Could you check a few things on this model? Use its own coordinates, in mm. Round coordinates to 2 decimals unless told otherwise and drop trailing zeros. Loops run counter-clockwise (first coordinate to the right, second up) from the corner with the lowest first, then second, coordinate; pieces in that order, holes last. Notation, with made-up numbers: (83, 4) -> (133, 4) arc R18 ccw to (133, 25) -> close; hole circle Ø6 at (-39, -39). An arc over 180 degrees is marked (long way). One line per item, written item: value.
```python
from build123d import *

# Parameters (mm, degrees)
BOSS_EXTRUDE1_DEPTH     = 1.5875
SKETCH2_R               = 0.635
CUT_EXTRUDE1_DEPTH      = 1
CUT_EXTRUDE1_DEPTH_BACK = 2.5875


with BuildPart() as part:
    # Sketch1 → Boss-Extrude1 (new body)
    with BuildSketch(Plane(origin=(0, 0, 0), x_dir=(1, 0, 0), z_dir=(0, 1, 0))):
        with BuildLine():
            Line((8.89, -66.675), (43.815, -66.675))
            Line((43.815, -66.675), (43.815, -1.27))
            ThreePointArc((43.815, -1.27), (43.453523156, -0.361476844), (42.545, 0))
            Line((42.545, 0), (-42.545, 0))
            Line((-42.545, 0), (-42.545, -57.785))
            Line((-42.545, -57.785), (-5.08, -57.785))
            ThreePointArc((-5.08, -57.785), (-4.181974388, -58.156974388), (-3.81, -59.055))
            ThreePointArc((-3.81, -59.055), (-3.438025612, -59.953025612), (-2.54, -60.325))
            Line((-2.54, -60.325), (2.54, -60.325))
            Line((2.54, -60.325), (2.54, -73.025))
            ThreePointArc((2.54, -73.025), (4.399871939, -68.534871939), (8.89, -66.675))
        make_face()
    extrude(amount=BOSS_EXTRUDE1_DEPTH)

    # Sketch2 → Cut-Extrude1 (cut, two sides)
    with BuildSketch(Plane(origin=(0, 1.5875, 0), x_dir=(-1, 0, 0), z_dir=(0, 1, 0))) as cut_extrude1_sk:
        with Locations((39.37, 3.175)):
            Circle(SKETCH2_R)
        with Locations((26.035, 3.175)):
            Circle(SKETCH2_R)
        with Locations((12.7, 3.175)):
            Circle(SKETCH2_R)
        with Locations((-0.635, 3.175)):
            Circle(SKETCH2_R)
        with Locations((-13.97, 3.175)):
            Circle(SKETCH2_R)
        with Locations((-27.305, 3.175)):
            Circle(SKETCH2_R)
        with Locations((-40.64, 3.175)):
            Circle(SKETCH2_R)
        with Locations((39.37, 16.03375)):
            Circle(SKETCH2_R)
        with Locations((39.37, 28.8925)):
            Circle(SKETCH2_R)
        with Locations((39.37, 41.75125)):
            Circle(SKETCH2_R)
        with Locations((-40.64, 15.24)):
            Circle(SKETCH2_R)
        with Locations((-40.64, 27.305)):
            Circle(SKETCH2_R)
        with Locations((-40.64, 39.37)):
            Circle(SKETCH2_R)
        with Locations((-40.64, 51.435)):
            Circle(SKETCH2_R)
        with Locations((-40.64, 63.5)):
            Circle(SKETCH2_R)
        with Locations((-24.994404736, 63.5)):
            Circle(SKETCH2_R)
        with Locations((-9.348809473, 63.5)):
            Circle(SKETCH2_R)
        with Locations((-1.889213751, 54.61)):
            Circle(SKETCH2_R)
        with Locations((11.863857499, 54.61)):
            Circle(SKETCH2_R)
        with Locations((25.61692875, 54.61)):
            Circle(SKETCH2_R)
        with Locations((39.37, 54.61)):
            Circle(SKETCH2_R)
    extrude(amount=CUT_EXTRUDE1_DEPTH, mode=Mode.SUBTRACT)
    extrude(cut_extrude1_sk.sketch, amount=-CUT_EXTRUDE1_DEPTH_BACK, mode=Mode.SUBTRACT)


solid = part.part
```
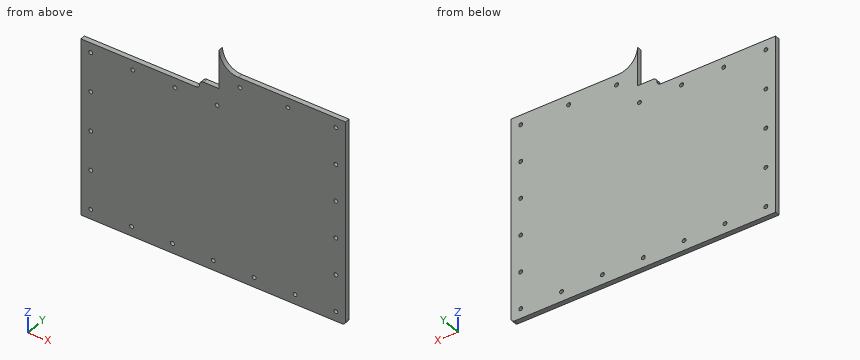
(1) Imagine slicing it at B-B on z = 68. Write out the boundary of the cut face in (x, y).
Results below:
outline: (2.54, 0) -> (5.01, 0) -> (5.01, 1.59) -> (2.54, 1.59) -> close
(2) Please list where these lines run through material, in increasing order: L1, parallel to X at y = 1.1, z = 54.61 (3 decimals); L2, parallel to Z at x = -39.37, y = 0.5 (1 decimal); L3, parallel to Z at x = 30, y = 1.3 (3 decimals).
Results below:
L1: x = -42.545 to -40.005, -38.735 to -26.252, -24.982 to -12.499, -11.229 to 1.254, 2.524 to 43.815
L2: z = 0 to 2.5, 3.8 to 15.4, 16.7 to 28.3, 29.5 to 41.1, 42.4 to 54, 55.2 to 57.8
L3: z = 0 to 66.675
(3) Imagine slicing it at A-A on y = 1.3. Give the number of separate pieces and of enclosed holes in the cut face, then the cut area to 3 significant figures.
Results below:
separate pieces: 1
enclosed holes: 21
area: 5,360 mm²
(4) Imagine slicing it at C-C on x = 20.5. Write out the boundary of the cut face in (y, z) (1 decimal).
Results below:
outline: (0, 0) -> (1.6, 0) -> (1.6, 66.7) -> (0, 66.7) -> close
(5) For pin 1 Ø0.8 at (x, y) = (0, 0.5) entering from +Z (3 decimals), with a flat end and sliding along its axis, tell me the tip position at first contact or that it passes through.
Results below:
pin 1: stops at z = 60.325
